Verification items for the finished model (mm, model axes). Give positions to 0.01 mm unless a question says otherwise; leave off trailing zeros. Write each loop counter-clockwise with the first axis right and the second up, starting at its lowest first coordinate (ties: lowest second). Pieces come first, ordered by that corner, then holes. Notation, with made-up numbers: (-1, -13) -> (22, -13) arc R23 ccw to (22, 2) -> close; hole circle Ø4 at (-34, -30). An arc over 180 degrees is marked (long way). Answer as CSV lines item,"result". Start each with the question number.
1) Sectioned sample at D-D on x = -60. Record the cut outline in (y, z).
2) Sectioned sample at A-A on x = 70.5. Record the cut outline in (y, z), and give its area (3 significant figures).
3) Sectioned sample at B-B on y = 0. Record the cut outline in (x, z), and give its area (3 significant figures).
4) Gauge pin test, flat end, axial feed: pin 1 Ø5 at (x, y) = (-60, 0) entering from -Z. Record the tip position at first contact, or that the pin passes through.
5) Sectioned sample at C-C on z = 1.4. Record the cut outline in (x, y).
6) Material ranges on L1, parallel to Y at x = -60, z = 1.85; L2, parallel to Y at x = 70.5, z = 2.1; L3, parallel to X at y = -2, z = 3.3, recorded low to high.
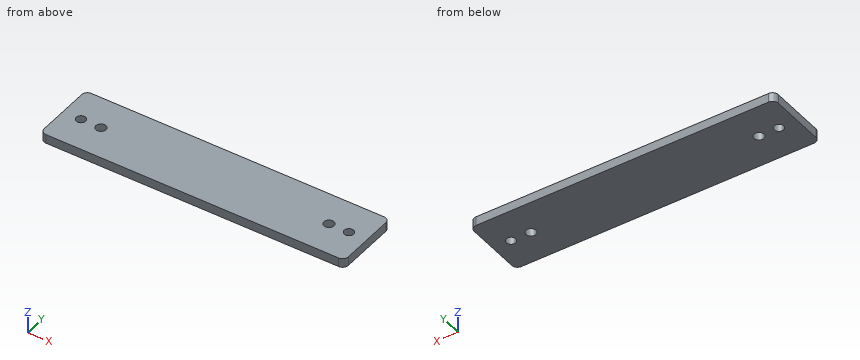
```python
from build123d import *

# Parameters (mm, degrees)
SKETCH1_W            = 160
SKETCH1_H            = 35
SKETCH1_R            = 2.5
BOSS_EXTRUDE1_DEPTH  = 4.7625
M5_CLEARANCE_HOLE1_D = 5.3
FILLET1_R            = 3


with BuildPart() as part:
    # Sketch1 → Boss-Extrude1 (new body)
    with BuildSketch(Plane.XY):
        Rectangle(SKETCH1_W, SKETCH1_H)
        with Locations(Location((-70.5, 0, 0), (0, 0, 180))):
            Circle(SKETCH1_R, mode=Mode.SUBTRACT)
        with Locations(Location((70.5, 0, 0), (0, 0, 180))):
            Circle(SKETCH1_R, mode=Mode.SUBTRACT)
    extrude(amount=BOSS_EXTRUDE1_DEPTH)

    # M5 Clearance Hole1 (through all)
    with Locations(Plane.XY.offset(4.7625)):
        with Locations((-60, 0), (60, 0)):
            Hole(M5_CLEARANCE_HOLE1_D / 2)

    # Fillet1
    fillet1_edges = [part.edges().sort_by_distance(p)[0] for p in [
        (80, -17.5, 2.38125),
        (-80, -17.5, 2.38125),
        (-80, 17.5, 2.38125),
        (80, 17.5, 2.38125),
    ]]
    fillet(fillet1_edges, radius=FILLET1_R)


solid = part.part
```
Ans:
1,outline,"(-17.5, 0) -> (-2.65, 0) -> (-2.65, 4.76) -> (-17.5, 4.76) -> close; (2.65, 0) -> (17.5, 0) -> (17.5, 4.76) -> (2.65, 4.76) -> close"
2,outline,"(-17.5, 0) -> (-2.5, 0) -> (-2.5, 4.76) -> (-17.5, 4.76) -> close; (2.5, 0) -> (17.5, 0) -> (17.5, 4.76) -> (2.5, 4.76) -> close"
2,area,"143 mm²"
3,outline,"(-80, 0) -> (-73, 0) -> (-73, 4.76) -> (-80, 4.76) -> close; (-68, 0) -> (-62.65, 0) -> (-62.65, 4.76) -> (-68, 4.76) -> close; (-57.35, 0) -> (57.35, 0) -> (57.35, 4.76) -> (-57.35, 4.76) -> close; (62.65, 0) -> (68, 0) -> (68, 4.76) -> (62.65, 4.76) -> close; (73, 0) -> (80, 0) -> (80, 4.76) -> (73, 4.76) -> close"
3,area,"664 mm²"
4,pin 1,"passes through"
5,outline,"(-80, -14.5) arc R3 ccw to (-77, -17.5) -> (77, -17.5) arc R3 ccw to (80, -14.5) -> (80, 14.5) arc R3 ccw to (77, 17.5) -> (-77, 17.5) arc R3 ccw to (-80, 14.5) -> close; hole circle Ø5 at (-70.5, 0); hole circle Ø5.3 at (-60, 0); hole circle Ø5.3 at (60, 0); hole circle Ø5 at (70.5, 0)"
6,L1,"y = -17.5 to -2.65, 2.65 to 17.5"
6,L2,"y = -17.5 to -2.5, 2.5 to 17.5"
6,L3,"x = -80 to -72, -69 to -61.74, -58.26 to 58.26, 61.74 to 69, 72 to 80"
